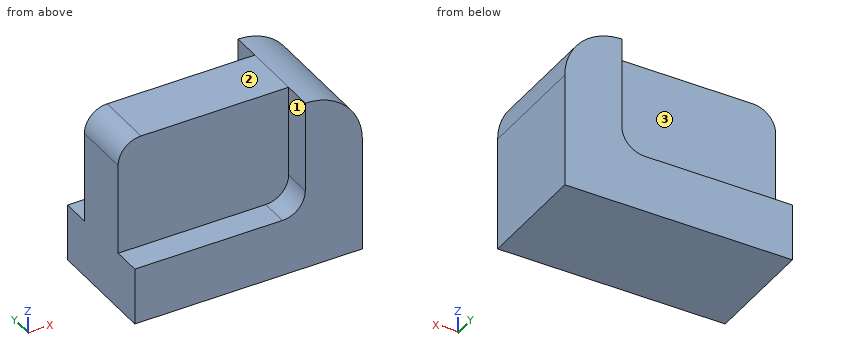
```python
from build123d import *

# Parameters (mm, degrees)
F1_DEPTH = 25.4
F2_W     = 37.8928769708
F2_H     = 6.35
F2_H_2   = 6.2968162
F3_DEPTH = 25.4
F4_R     = 5.08


with BuildPart() as f1:
    # F0 (on Front) → F1 (new body)
    with BuildSketch(Plane.XZ):
        with BuildLine():
            Line((-50.5928769708, 0), (0, 0))
            Line((0, 0), (0, 25.4))
            ThreePointArc((0, 25.4), (-3.7197438789, 34.3802561211), (-12.7, 38.1))
            Line((-12.7, 38.1), (-50.5928769708, 38.1))
            Line((-50.5928769708, 38.1), (-50.5928769708, 0))
        make_face()
    extrude(amount=F1_DEPTH)

    # F2 (on face) → F3 (cut)
    with BuildSketch(Plane.XY.offset(38.1)):
        with Locations((-31.6464384854, -3.175)):
            Rectangle(F2_W, F2_H)
        with Locations((-31.6464384854, -22.2515919)):
            Rectangle(F2_W, F2_H_2)
    extrude(amount=-F3_DEPTH, mode=Mode.SUBTRACT)

    # F4
    f4_edges = [f1.edges().sort_by_distance(p)[0] for p in [
        (-12.7, -22.251592, 12.7),
        (-12.7, -3.175, 12.7),
        (-50.592877, -12.726592, 38.1),
    ]]
    fillet(f4_edges, radius=F4_R)


solid = f1.part
```
For this review, take the finished solid that the model builds, in its own axes (mm). Face numbers are marked on the shaded views. A direction names the side the tool comes from. Round coordinates to 2 decimals unless told otherwise and drop trailing zeros. Write each loop counter-clockwise with the first axis right and the second up, starting at its lowest first coordinate (ties: lowest second). Pieces come first, ordered by that corner, then holes. Notation, with made-up numbers: (8, 19.25) -> (26, 19.25) arc R38 ccw to (26, 58.25) -> close; hole circle Ø4 at (52.5, 18.25). An arc over 180 degrees is marked (long way). One line per question, with ' | ' between items. Start each with the question number.
1) Wall thickness on line 1 along Y through (x, z) = (-42.5, 20.5); line 2 along Z through (x, y) = (-46, -5.25); line 3 along X through (y, z) = (-9.75, 31): over which ranges is each line inside the solid? List them lowest first.
2) For pin 1 Ø1.9 at (x, y) = (-26.5, -23.5) entering from +Z; pin 2 Ø12.5 at (x, z) = (-25.5, 19.5) entering from -Y; pin 3 Ø3 at (y, z) = (-22.5, 29.5) entering from -X, all flat-tipped, find the tip position at first contact; note any pin that passes through.
3) Add section D-D (y = -3.5). Write out the cut boundary in (x, z).
4) Add section B-B (x = -24.5). Write out the cut boundary in (y, z), and give its area (3 significant figures).
5) Add section A-A (z = 21). Write out the cut boundary in (x, y).
6) Add section C-C (y = -11.5). Write out the cut boundary in (x, z).
7) Machinability: for the marked faces 1, 2 and 3, which of the approach directions +Z, -Z, +X, -X, +Y, -Y give a long, thin tool a straight path to every point of the face, cutting with its end or side? Answer none if there is none.
Reported:
1) line 1: y = -19.1 to -6.35 | line 2: z = 0 to 12.7 | line 3: x = -50.59 to -1.3
2) pin 1: stops at z = 12.7 | pin 2: stops at y = -19.1 | pin 3: stops at x = -12.7
3) outline: (-50.59, 0) -> (0, 0) -> (0, 25.4) arc R12.7 ccw to (-12.7, 38.1) -> (-12.7, 17.78) arc R5.08 cw to (-17.78, 12.7) -> (-50.59, 12.7) -> close
4) outline: (-25.4, 0) -> (0, 0) -> (0, 12.7) -> (-6.35, 12.7) -> (-6.35, 38.1) -> (-19.1, 38.1) -> (-19.1, 12.7) -> (-25.4, 12.7) -> close | area: 647 mm²
5) outline: (-50.59, -19.1) -> (-12.7, -19.1) -> (-12.7, -25.4) -> (0, -25.4) -> (0, 0) -> (-12.7, 0) -> (-12.7, -6.35) -> (-50.59, -6.35) -> close
6) outline: (-50.59, 0) -> (0, 0) -> (0, 25.4) arc R12.7 ccw to (-12.7, 38.1) -> (-45.51, 38.1) arc R5.08 ccw to (-50.59, 33.02) -> close
7) face 1: +Z, -X, -Y | face 2: +Z, +X, -X, +Y, -Y | face 3: +Z, -X, +Y
